Input: part model. Units: mm. Frame: model coordinates. A direction names the side the tool comes from. Coordinates: 2 decimals unless noted, no trailing zeros. Loops run counter-clockwise (first coordinate to the right, second up) from the corner with the lowest first, then second, coordinate; pieces in that order, holes last.
(1) Section B-B, the plane x = -13. Return loops of the section in (y, z), then the cut area to 3 significant figures.
(2) Set-up query: faces 1 (the face through (21, 5, -9.05)), 2 (the face through (21, 5, -11.05)), 3 (the face through (-18.9, 2, -5)), 4 (the face through (20.1, 5, -10)). Return all of +Z, -Z, +X, -X, +Y, -Y with unobstructed straight access to the full face (end or side cutting, diameter ignored); none if empty.
(3) Section A-A, the plane y = 7. Return loops of the section in (x, z).
(4) Line query: L1, parallel to X at y = 3.25, z = 9.5; L2, parallel to X at y = 1, z = 2.5; L3, parallel to Z at x = -11.5, y = 1.5. Output: solid intervals per line, ascending.
(5) Section C-C, the plane y = 0.75. Return loops of the section in (x, z).
(6) Mould query, pull axis X, two halves, no side actions, for faces 5 (the face through (-14, 2, 2.65)), 6 (the face through (-22.1, 5, -10)), 7 (the face through (0, 0, 0)). Classes: released by +X, released by -X, zero draft, split by the parting line, or undercut.
(7) Contact query for flat-ended pins moving along their axis: P1, Ø2, axis at y = 6.5, z = 10.5, coming from the +X side; P2, Ø1, axis at y = 6, z = -10, coming from the -X side; P3, Ø1.6, axis at x = 21.5, y = 4.5, coming from the -Z side; P4, Ø2, axis at x = -17.5, z = -4, coming from the +Y side. Output: stop coordinate, or through.
(8) Section D-D, the plane z = -4.5. Return loops of the section in (x, y).
```python
from build123d import *

# Parameters (mm, degrees)
SCHIZZO1_W                   = 47.8
SCHIZZO1_H                   = 25.7
ESTRUSIONE_ESTRUSIONE2_DEPTH = 3.2
SCHIZZO3_W                   = 2
SCHIZZO3_H                   = 2
ESTRUSIONE_ESTRUSIONE4_DEPTH = 4.5
SCHIZZO4_W                   = 10
SCHIZZO4_H                   = 14.5
TAGLIO_ESTRUSIONE1_DEPTH     = 5


with BuildPart() as part:
    # Schizzo1 → Estrusione-Estrusione2 (new body)
    with BuildSketch(Plane(origin=(0, 0, 0), x_dir=(1, 0, 0), z_dir=(0, 1, 0))):
        Rectangle(SCHIZZO1_W, SCHIZZO1_H)
    extrude(amount=ESTRUSIONE_ESTRUSIONE2_DEPTH)

    # Schizzo3 → Estrusione-Estrusione4 (add)
    with BuildSketch(Plane(origin=(0, 3.2, 0), x_dir=(1, 0, 0), z_dir=(0, 1, 0))):
        with Locations((21.1, -10.05)):
            Rectangle(SCHIZZO3_W, SCHIZZO3_H)
        with Locations((21.1, 10.05)):
            Rectangle(SCHIZZO3_W, SCHIZZO3_H)
        with Locations((-21.1, 10.05)):
            Rectangle(SCHIZZO3_W, SCHIZZO3_H)
        with Locations((-21.1, -10.05)):
            Rectangle(SCHIZZO3_W, SCHIZZO3_H)
    extrude(amount=ESTRUSIONE_ESTRUSIONE4_DEPTH)

    # Schizzo4 → Taglio-Estrusione1 (cut)
    with BuildSketch(Plane.XZ):
        with Locations((-13.9, -4.6)):
            Rectangle(SCHIZZO4_W, SCHIZZO4_H)
    extrude(amount=-TAGLIO_ESTRUSIONE1_DEPTH, mode=Mode.SUBTRACT)


solid = part.part
```
Report:
1. outline: (0, -12.85) - (3.2, -12.85) - (3.2, -11.85) - (0, -11.85) - close; (0, 2.65) - (3.2, 2.65) - (3.2, 12.85) - (0, 12.85) - close
1. area: 35.8 mm2
2. face 1: +X, -X, +Y
2. face 2: -Z, +X, -X, +Y
2. face 3: +Y, -Y
2. face 4: +Z, -Z, +Y
3. outline: (-22.1, -11.05) - (-20.1, -11.05) - (-20.1, -9.05) - (-22.1, -9.05) - close; (-22.1, 9.05) - (-20.1, 9.05) - (-20.1, 11.05) - (-22.1, 11.05) - close; (20.1, -11.05) - (22.1, -11.05) - (22.1, -9.05) - (20.1, -9.05) - close; (20.1, 9.05) - (22.1, 9.05) - (22.1, 11.05) - (20.1, 11.05) - close
4. L1: x = -22.1 to -20.1, 20.1 to 22.1
4. L2: x = -23.9 to -18.9, -8.9 to 23.9
4. L3: z = -12.85 to -11.85, 2.65 to 12.85
5. outline: (-23.9, -12.85) - (23.9, -12.85) - (23.9, 12.85) - (-23.9, 12.85) - close; hole (-18.9, -11.85) - (-8.9, -11.85) - (-8.9, 2.65) - (-18.9, 2.65) - close
6. face 5: undercut
6. face 6: released by -X
6. face 7: zero draft
7. P1: stops at x = 22.1
7. P2: stops at x = -22.1
7. P3: stops at z = -11.05
7. P4: passes through
8. outline: (-23.9, 0) - (-18.9, 0) - (-18.9, 3.2) - (-23.9, 3.2) - close; (-8.9, 0) - (23.9, 0) - (23.9, 3.2) - (-8.9, 3.2) - close
